from build123d import *

# Parameters (mm, degrees)
F0_R     = 7.5
F1_DEPTH = 2
F2_R     = 5.9
F3_DEPTH = 4.3
F4_R     = 1.65
F5_DEPTH = 6.301
F6_SIZE  = 0.5


with BuildPart() as f1:
    # F0 (on Top) → F1 (new body)
    with BuildSketch(Plane.XY):
        Circle(F0_R)
    extrude(amount=F1_DEPTH)

    # F2 (on face) → F3 (join)
    with BuildSketch(Plane.XY.offset(2)):
        Circle(F2_R)
    extrude(amount=F3_DEPTH)

    # F4 (on face) → F5 (cut, through all)
    with BuildSketch(Plane.XY.offset(6.3)):
        Circle(F4_R)
    extrude(amount=-F5_DEPTH, mode=Mode.SUBTRACT)

    # F6
    f6_edges = [f1.edges().sort_by_distance(p)[0] for p in [
        (-5.9, 0, 6.3),
    ]]
    chamfer(f6_edges, length=F6_SIZE)


solid = f1.part
Part model, mm, in its own coordinate system. A direction names the side the tool comes from. Give positions to 0.01 mm unless a question says otherwise; leave off trailing zeros. Write each loop counter-clockwise with the first axis right and the second up, starting at its lowest first coordinate (ties: lowest second). Pieces come first, ordered by that corner, then holes.
1) Probe L1, parallel to Y at x = 0, z = 2.75; L2, parallel to Y at x = 0, z = 1.5; L3, parallel to Z at x = 1.5, y = 6. List the from-to ranges inside material, lowest first.
Resolved:
L1: y = -5.9 to -1.65, 1.65 to 5.9
L2: y = -7.5 to -1.65, 1.65 to 7.5
L3: z = 0 to 2
2) Cut at D-D on y = -6.5. Write the cut outline in (x, z), then the cut area to 3 significant figures.
Resolved:
outline: (-3.74, 0) - (3.74, 0) - (3.74, 2) - (-3.74, 2) - close
area: 15.0 mm2
3) Cut at C-C on z = 5.25. Write the cut outline in (x, y), then the cut area to 3 significant figures.
Resolved:
outline: circle Ø11.8 at (0, 0); hole circle Ø3.3 at (0, 0)
area: 101 mm2
4) Which spindle directions (+Z, -Z, +X, -X, +Y, -Y) get a long thin tool onto all of the face, cutting with end or side? Do faces 1 (the face through (-5.894, 0.259, 3.873)), 2 (the face through (-1.3, 1.3, 6.3)). Say none if no direction does.
Resolved:
face 1: +Z
face 2: +Z, +X, -X, +Y, -Y
5) Pin check, flat tips, straight feed: pin 1 (2 mm diameter, centred on x = -5, y = -3, fed in from +Z); pin 2 (2.5 mm diameter, centred on x = 0, y = 0, fed in from +Z); pin 3 (1.5 mm diameter, centred on y = 3, z = 4.5, fed in from +X). Stop position of each tip, or through.
Resolved:
pin 1: stops at z = 6.3
pin 2: passes through
pin 3: stops at x = 5.45
6) Cut at A-A on y = 0. Write the cut outline in (x, z), then the cut area to 3 significant figures.
Resolved:
outline: (-7.5, 0) - (-1.65, 0) - (-1.65, 6.3) - (-5.4, 6.3) - (-5.9, 5.8) - (-5.9, 2) - (-7.5, 2) - close; (1.65, 0) - (7.5, 0) - (7.5, 2) - (5.9, 2) - (5.9, 5.8) - (5.4, 6.3) - (1.65, 6.3) - close
area: 59.7 mm2
7) Two-plate mould, pull along X, no slides. Class faces 3 (the face through (-7.493, 0.33, 0.986)), 4 (the face through (-1.216, 1.115, 3.194)), 5 (the face through (0, 2, 0)): released by +X, released by -X, zero draft, split by the parting line, or undercut.
Resolved:
face 3: split by the parting line
face 4: undercut
face 5: zero draft
